Can you work these out from the model? Positions are in its coordinate system, mm. Face numbers are marked on the shaded views. A direction names the side the tool comes from. Give positions to 0.01 mm unless a question says otherwise; leave off trailing zeros. Order: outer loops, then holes, each group sorted by start corner. A loop starts at its lowest first (then second) coordinate and runs counter-clockwise, first axis right, second up. Notation, with made-up numbers: (78, 73) - (88, 73) arc R20 ccw to (88, 97) - close; hole circle Ø5 at (81, 76). An arc over 180 degrees is marked (long way). Answer as CSV lines item,"result".
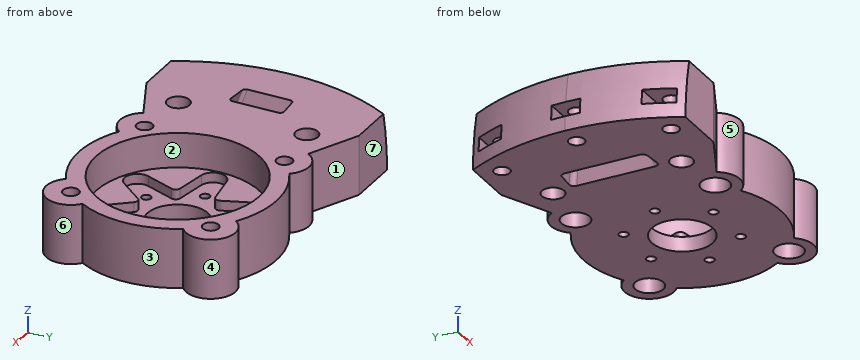
```python
from build123d import *

# Parameters (mm, degrees)
PAD_DEPTH       = 12
SKETCH001_R     = 1.6
POCKET_DEPTH    = 12.001
SKETCH006_R     = 2.85
POCKET005_DEPTH = 8
SKETCH002_R     = 16.5
POCKET001_DEPTH = 7
SKETCH003_R     = 6.15
POCKET002_DEPTH = 12.001
POCKET003_DEPTH = 2
SKETCH005_R     = 0.95
POCKET004_DEPTH = 12.001
SKETCH007_R     = 2.25
POCKET006_DEPTH = 12.001
SKETCH008_R     = 1.6
POCKET007_DEPTH = 8
SKETCH009_W     = 11
SKETCH009_H     = 5.8
POCKET008_DEPTH = 3
GROOVE_ANGLE    = 90
CHAMFER_1_ANGLE = 45
CHAMFER_1_SIZE  = 1.2
CHAMFER_2_ANGLE = 45
CHAMFER_2_SIZE  = 1.2
CHAMFER_3_ANGLE = 45
CHAMFER_3_SIZE  = 1.2
CHAMFER_4_ANGLE = 45
CHAMFER_4_SIZE  = 1.2


with BuildPart() as part:
    # Sketch → Pad (new body)
    with BuildSketch(Plane.XY):
        with BuildLine():
            ThreePointArc((10.19239, 17.207998), (0, 20), (-10.19239, 17.207998))
            ThreePointArc((-10.19239, 17.207998), (-14.460107, 19.132015), (-18.449087, 16.681855))
            Line((-28.781633, 21.5), (-18.449087, 16.681855))
            Line((-28.781633, 21.5), (-39.531633, 21.5))
            ThreePointArc((-39.531633, 21.5), (-45, 0), (-39.531633, -21.5))
            Line((-39.531633, -21.5), (-28.781633, -21.5))
            Line((-28.781633, -21.5), (-18.449087, -16.681855))
            ThreePointArc((-18.449087, -16.681855), (-14.460107, -19.132015), (-10.19239, -17.207998))
            ThreePointArc((-10.19239, -17.207998), (0, -20), (10.19239, -17.207998))
            ThreePointArc((10.19239, -17.207998), (17.67767, -17.67767), (17.207998, -10.19239))
            ThreePointArc((17.207998, -10.19239), (20, 0), (17.207998, 10.19239))
            ThreePointArc((17.207998, 10.19239), (17.67767, 17.67767), (10.19239, 17.207998))
        make_face()
    extrude(amount=PAD_DEPTH)

    # Sketch001 → Pocket (cut, through all)
    with BuildSketch(Plane.XY):
        with Locations((-14.142136, 14.142136)):
            Circle(SKETCH001_R)
        with Locations((14.142136, 14.142136)):
            Circle(SKETCH001_R)
        with Locations((14.142136, -14.142136)):
            Circle(SKETCH001_R)
        with Locations((-14.142136, -14.142136)):
            Circle(SKETCH001_R)
    extrude(amount=POCKET_DEPTH, mode=Mode.SUBTRACT)

    # Sketch006 → Pocket005 (cut)
    with BuildSketch(Plane.XY):
        with Locations((-14.142136, 14.142136)):
            Circle(SKETCH006_R)
        with Locations((14.142136, 14.142136)):
            Circle(SKETCH006_R)
        with Locations((14.142136, -14.142136)):
            Circle(SKETCH006_R)
        with Locations((-14.142136, -14.142136)):
            Circle(SKETCH006_R)
    extrude(amount=POCKET005_DEPTH, mode=Mode.SUBTRACT)

    # Sketch002 → Pocket001 (cut)
    with BuildSketch(Plane.XY.offset(12)):
        Circle(SKETCH002_R)
    extrude(amount=-POCKET001_DEPTH, mode=Mode.SUBTRACT)

    # Sketch003 → Pocket002 (cut, through all)
    with BuildSketch(Plane.XY):
        Circle(SKETCH003_R)
    extrude(amount=POCKET002_DEPTH, mode=Mode.SUBTRACT)

    # Sketch004 → Pocket003 (cut)
    with BuildSketch(Plane.XY.offset(5)):
        with BuildLine():
            ThreePointArc((9.178305, 10.762186), (8.05, 13.943009), (4.731174, 13.329739))
            Line((4.731174, 13.329739), (0.776472, 8.456766))
            ThreePointArc((-0.776472, 8.456766), (0, 8.086918), (0.776472, 8.456766))
            Line((-0.776472, 8.456766), (-4.731174, 13.329739))
            ThreePointArc((-4.731174, 13.329739), (-8.05, 13.943009), (-9.178305, 10.762186))
            Line((-9.178305, 10.762186), (-6.935538, 4.900827))
            ThreePointArc((-7.71201, 3.555939), (-7.003477, 4.043459), (-6.935538, 4.900827))
            Line((-7.71201, 3.555939), (-13.909479, 2.567553))
            ThreePointArc((-13.909479, 2.567553), (-16.1, 0), (-13.909479, -2.567553))
            Line((-13.909479, -2.567553), (-7.71201, -3.555939))
            ThreePointArc((-6.935538, -4.900827), (-7.003477, -4.043459), (-7.71201, -3.555939))
            Line((-6.935538, -4.900827), (-9.178305, -10.762186))
            ThreePointArc((-9.178305, -10.762186), (-8.05, -13.943009), (-4.731174, -13.329739))
            Line((-0.776472, -8.456766), (-4.731174, -13.329739))
            ThreePointArc((0.776472, -8.456766), (0, -8.086918), (-0.776472, -8.456766))
            Line((0.776472, -8.456766), (4.731174, -13.329739))
            ThreePointArc((4.731174, -13.329739), (8.05, -13.943009), (9.178305, -10.762186))
            Line((9.178305, -10.762186), (6.935538, -4.900827))
            ThreePointArc((7.71201, -3.555939), (7.003477, -4.043459), (6.935538, -4.900827))
            Line((7.71201, -3.555939), (13.909479, -2.567553))
            ThreePointArc((13.909479, -2.567553), (16.1, 0), (13.909479, 2.567553))
            Line((13.909479, 2.567553), (7.71201, 3.555939))
            ThreePointArc((6.935538, 4.900827), (7.003477, 4.043459), (7.71201, 3.555939))
            Line((6.935538, 4.900827), (9.178305, 10.762186))
        make_face()
    extrude(amount=-POCKET003_DEPTH, mode=Mode.SUBTRACT)

    # Sketch005 → Pocket004 (cut, through all)
    with BuildSketch(Plane.XY):
        with Locations((5.25, 9.093267)):
            Circle(SKETCH005_R)
        with Locations((10.5, 0)):
            Circle(SKETCH005_R)
        with Locations((-5.25, 9.093267)):
            Circle(SKETCH005_R)
        with Locations((-10.5, 0)):
            Circle(SKETCH005_R)
        with Locations((-5.25, -9.093267)):
            Circle(SKETCH005_R)
        with Locations((5.25, -9.093267)):
            Circle(SKETCH005_R)
    extrude(amount=POCKET004_DEPTH, mode=Mode.SUBTRACT)

    # Sketch007 → Pocket006 (cut, through all)
    with BuildSketch(Plane.XY):
        with Locations((-24.9, 13)):
            Circle(SKETCH007_R)
        with Locations((-24.9, -13)):
            Circle(SKETCH007_R)
    extrude(amount=POCKET006_DEPTH, mode=Mode.SUBTRACT)

    # Sketch008 → Pocket007 (cut)
    with BuildSketch(Plane.XY):
        with Locations((-40.5, 0)):
            Circle(SKETCH008_R)
        with Locations((-36.705465, 17.11604)):
            Circle(SKETCH008_R)
        with Locations((-36.705465, -17.11604)):
            Circle(SKETCH008_R)
    extrude(amount=POCKET007_DEPTH, mode=Mode.SUBTRACT)

    # Sketch009 → Pocket008 (cut)
    with BuildSketch(Plane.XY.offset(3)):
        with Locations((-42.8, 0)):
            Rectangle(SKETCH009_W, SKETCH009_H)
        with Locations((-39.005465, 17.11604)):
            Rectangle(SKETCH009_W, SKETCH009_H)
        with Locations((-39.005465, -17.11604)):
            Rectangle(SKETCH009_W, SKETCH009_H)
    extrude(amount=POCKET008_DEPTH, mode=Mode.SUBTRACT)

    # Sketch010 → SubtractiveLoft section 0
    with BuildSketch(Plane.XY):
        with BuildLine():
            Line((-30.7, -7.628728), (-30.7, 7.628728))
            ThreePointArc((-29.787156, 8.624922), (-30.437277, 8.304318), (-30.7, 7.628728))
            Line((-29.787156, 8.624922), (-26.587156, 8.904886))
            ThreePointArc((-25.5, 7.908691), (-25.82441, 8.645969), (-26.587156, 8.904886))
            Line((-25.5, 7.908691), (-25.5, -7.908691))
            ThreePointArc((-26.587156, -8.904886), (-25.82441, -8.645969), (-25.5, -7.908691))
            Line((-26.587156, -8.904886), (-29.787156, -8.624922))
            ThreePointArc((-30.7, -7.628728), (-30.437277, -8.304318), (-29.787156, -8.624922))
        make_face()
    # Sketch011 → SubtractiveLoft section 1
    with BuildSketch(Plane.XY.offset(12)):
        with BuildLine():
            Line((-35, 4.312752), (-35, -4.312752))
            ThreePointArc((-35, -4.312752), (-34.802958, -4.819444), (-34.315367, -5.059898))
            Line((-34.315367, -5.059898), (-30.615367, -5.383606))
            ThreePointArc((-30.615367, -5.383606), (-30.043307, -5.189418), (-29.8, -4.63646))
            Line((-29.8, -4.63646), (-29.8, 4.63646))
            ThreePointArc((-29.8, 4.63646), (-30.043307, 5.189418), (-30.615367, 5.383606))
            Line((-30.615367, 5.383606), (-34.315367, 5.059898))
            ThreePointArc((-34.315367, 5.059898), (-34.802958, 4.819444), (-35, 4.312752))
        make_face()
    loft(mode=Mode.SUBTRACT)

    # Sketch012 → Groove (revolve, symmetric, cut)
    with BuildSketch(Plane.XZ) as groove_sk:
        with BuildLine():
            Line((-45, 0), (-45, 12))
            Line((-45, 12), (-43.787754, 12))
            ThreePointArc((-43.787754, 12), (-44.696169, 6.030538), (-45, 0))
        make_face()
    revolve(axis=Axis((0, 0, 0), (0, 0, 1)), revolution_arc=GROOVE_ANGLE / 2, mode=Mode.SUBTRACT)
    revolve(groove_sk.sketch, axis=Axis((0, 0, 0), (0, 0, -1)), revolution_arc=GROOVE_ANGLE / 2, mode=Mode.SUBTRACT)

    # Chamfer 1
    chamfer_1_edges = [part.edges().sort_by_distance(p)[0] for p in [
        (-15.742136, 14.142136, 8),
    ]]
    chamfer_1_side = part.faces().sort_by_distance((-15.742136, 14.142136, 10))[0]
    chamfer(chamfer_1_edges, length=CHAMFER_1_SIZE, angle=CHAMFER_1_ANGLE, reference=chamfer_1_side)

    # Chamfer 2
    chamfer_2_edges = [part.edges().sort_by_distance(p)[0] for p in [
        (12.542136, 14.142136, 8),
    ]]
    chamfer_2_side = part.faces().sort_by_distance((12.542136, 14.142136, 10))[0]
    chamfer(chamfer_2_edges, length=CHAMFER_2_SIZE, angle=CHAMFER_2_ANGLE, reference=chamfer_2_side)

    # Chamfer 3
    chamfer_3_edges = [part.edges().sort_by_distance(p)[0] for p in [
        (12.542136, -14.142136, 8),
    ]]
    chamfer_3_side = part.faces().sort_by_distance((12.542136, -14.142136, 10))[0]
    chamfer(chamfer_3_edges, length=CHAMFER_3_SIZE, angle=CHAMFER_3_ANGLE, reference=chamfer_3_side)

    # Chamfer 4
    chamfer_4_edges = [part.edges().sort_by_distance(p)[0] for p in [
        (-15.742136, -14.142136, 8),
    ]]
    chamfer_4_side = part.faces().sort_by_distance((-15.742136, -14.142136, 10))[0]
    chamfer(chamfer_4_edges, length=CHAMFER_4_SIZE, angle=CHAMFER_4_ANGLE, reference=chamfer_4_side)


solid = part.part
```
1) I'm going to push flat-ended pins straight in: P1, Ø3, axis at x = -2, y = -3.5, coming from the +Z side; P2, Ø0.9, axis at y = 16.5, z = 5, coming from the -X side; P3, Ø2.5, axis at x = -5.25, y = -9.09, coming from the +Z side; P4, Ø23, axis at x = -2, y = 1.5, coming from the +Z side. Where does each tip first touch, or does it pass through?
Answer block:
P1,"through"
P2,"x = -33.51"
P3,"z = 3"
P4,"z = 5"
2) If we mould it in two halves opening along Y, with no side actions, what happens to the marked faces 4, 5, 6 and 7? For each: +Y half, -Y half, draft (parallel to the pull), parting line (faces both ways), or undercut.
Answer block:
face 4,"undercut"
face 5,"-Y half"
face 6,"undercut"
face 7,"+Y half"
3) I need wall thicknesses on line 1 along Y through (x, z) = (-35, 4.5); line 2 along Z through (x, y) = (-40, -15); line 3 along Y through (x, z) = (-40, 4.25). Which ranges of each line are inside material? Lowest first, please. Write a range as [from, to].
Answer block:
line 1,"[-21.5, -20.02], [-14.22, 14.22], [20.02, 21.5]"
line 2,"[0, 3], [6, 12]"
line 3,"[-20.28, -20.02], [-14.22, -2.9], [2.9, 14.22], [20.02, 20.28]"
4) Which directions (+Z, -Z, +X, -X, +Y, -Y) give clear straight access to the entire face, cutting with the end or side of a thin tool? Please do the marked faces 1, 2 and 3.
Answer block:
face 1,"+Z, -Z, +Y"
face 2,"+Z"
face 3,"+Z, -Z, +X"
5) I want a section at A-A on x = 0. Write out the boundary of the cut face in (y, z), plus the area to 3 significant figures.
Answer block:
outline,"(-20, 0) - (-6.15, 0) - (-6.15, 3) - (-8.09, 3) - (-8.09, 5) - (-16.5, 5) - (-16.5, 12) - (-20, 12) - close; (6.15, 0) - (20, 0) - (20, 12) - (16.5, 12) - (16.5, 5) - (8.09, 5) - (8.09, 3) - (6.15, 3) - close"
area,"180 mm2"
6) I want a section at B-B on y = -18. Count the separate pieces of the cut face and the enclosed holes in it, plus the area to 3 significant figures.
Answer block:
separate pieces,"5"
enclosed holes,"0"
area,"560 mm2"
